Geometry: final body of the model. Coordinates: model frame, mm. Give positions to 0.01 mm unless a question says otherwise; leave off trailing zeros. Write each loop counter-clockwise with the first axis right and the second up, starting at its lowest first coordinate (ties: lowest second). Pieces come first, ordered by that corner, then holes. Notation, with made-up numbers: (23.25, 29) -> (47.25, 29) arc R21 cw to (47.25, 51) -> close; hole circle Ø6 at (85.25, 69). An arc over 180 degrees is marked (long way). Answer as a JSON object with one key per item and string values. Group by question number.
(1) Draft query along Z for faces 1 (the face through (3.13, -37.68, -101.61)), 2 (the face through (0, -166, -142)). Return one class per face: +Z half, -Z half, draft (parallel to the pull), parting line (faces both ways), or undercut.
(2) Material intervals for probe 1 along Y at (x, z) = (6, -158) (3 decimals); probe 2 along Z at (x, y) = (3.75, -44.5); probe 3 along Y at (x, z) = (6.25, -164.5) (3 decimals), sorted ascending.
(3) Contact query for flat-ended pins moving along their axis: pin 1 Ø1.9 at (x, z) = (2, 2) entering from -Y; pin 2 Ø1 at (x, z) = (3, -233) entering from +Y; pin 3 Ø3 at (x, y) = (4, -81) entering from -Z. Output: stop coordinate, or through.
(4) Section query C-C on y = -83. Output: boundary loops of the cut face in (x, z), plus the area to 3 significant figures.
(5) Section query B-B on z = -266. Output: boundary loops of the cut face in (x, y), plus the area to 3 significant figures.
(6) Section query A-A on x = 2.25. State how many separate pieces and enclosed holes the cut face has, plus the area to 3 significant figures.
from build123d import *

# Parameters (mm, degrees)
SKETCH1_R           = 9.525
SKETCH1_W           = 12.573
SKETCH1_H           = 6.35
BOSS_EXTRUDE1_DEPTH = 6.35


with BuildPart() as part:
    # Sketch1 → Boss-Extrude1 (new body)
    with BuildSketch(Plane(origin=(0, 0, 0), x_dir=(0, 0, -1), z_dir=(1, 0, 0))):
        Polygon((0, 0), (6.223, 0), (6.223, 6.35), (19.177, 6.35), (19.177, 0), (260.223, 0), (260.223, 6.35), (273.177, 6.35), (273.177, 0), (279.4, 0), (279.4, -12.573), (285.75, -12.573), (285.75, -25.527), (279.4, -25.527), (279.4, -37.973), (285.75, -37.973), (285.75, -50.927), (279.4, -50.927), (279.4, -63.373), (285.75, -63.373), (285.75, -76.327), (279.4, -76.327), (279.4, -88.773), (285.75, -88.773), (285.75, -101.727), (279.4, -101.727), (279.4, -114.173), (285.75, -114.173), (285.75, -127.127), (279.4, -127.127), (279.4, -139.573), (285.75, -139.573), (285.75, -152.527), (279.4, -152.527), (279.4, -164.973), (285.75, -164.973), (285.75, -177.927), (279.4, -177.927), (279.4, -190.373), (285.75, -190.373), (285.75, -203.327), (279.4, -203.327), (279.4, -215.773), (285.75, -215.773), (285.75, -228.727), (279.4, -228.727), (279.4, -241.173), (285.75, -241.173), (285.75, -254.127), (279.4, -254.127), (279.4, -266.573), (285.75, -266.573), (285.75, -279.527), (279.4, -279.527), (279.4, -291.973), (285.75, -291.973), (285.75, -304.927), (279.4, -304.927), (279.4, -317.373), (285.75, -317.373), (285.75, -330.327), (279.4, -330.327), (279.4, -342.9), (272.923, -342.9), (272.923, -336.55), (260.477, -336.55), (260.477, -342.9), (247.523, -342.9), (247.523, -336.55), (235.077, -336.55), (235.077, -342.9), (222.123, -342.9), (222.123, -336.55), (209.677, -336.55), (209.677, -342.9), (196.723, -342.9), (196.723, -336.55), (184.277, -336.55), (184.277, -342.9), (171.323, -342.9), (171.323, -336.55), (158.877, -336.55), (158.877, -342.9), (145.923, -342.9), (145.923, -336.55), (133.477, -336.55), (133.477, -342.9), (120.523, -342.9), (120.523, -336.55), (108.077, -336.55), (108.077, -342.9), (95.123, -342.9), (95.123, -336.55), (82.677, -336.55), (82.677, -342.9), (69.723, -342.9), (69.723, -336.55), (57.277, -336.55), (57.277, -342.9), (44.323, -342.9), (44.323, -336.55), (31.877, -336.55), (31.877, -342.9), (18.923, -342.9), (18.923, -336.55), (6.477, -336.55), (6.477, -342.9), (0, -342.9), (0, -330.327), (-6.35, -330.327), (-6.35, -317.373), (0, -317.373), (0, -304.927), (-6.35, -304.927), (-6.35, -291.973), (0, -291.973), (0, -279.527), (-6.35, -279.527), (-6.35, -266.573), (0, -266.573), (0, -254.127), (-6.35, -254.127), (-6.35, -241.173), (0, -241.173), (0, -228.727), (-6.35, -228.727), (-6.35, -215.773), (0, -215.773), (0, -203.327), (-6.35, -203.327), (-6.35, -190.373), (0, -190.373), (0, -177.927), (-6.35, -177.927), (-6.35, -164.973), (0, -164.973), (0, -152.527), (-6.35, -152.527), (-6.35, -139.573), (0, -139.573), (0, -127.127), (-6.35, -127.127), (-6.35, -114.173), (0, -114.173), (0, -101.727), (-6.35, -101.727), (-6.35, -88.773), (0, -88.773), (0, -76.327), (-6.35, -76.327), (-6.35, -63.373), (0, -63.373), (0, -50.927), (-6.35, -50.927), (-6.35, -37.973), (0, -37.973), (0, -25.527), (-6.35, -25.527), (-6.35, -12.573), (0, -12.573), align=None)
        with Locations((111.125, -38.1)):
            Circle(SKETCH1_R, mode=Mode.SUBTRACT)
        with Locations((168.275, -38.1)):
            Circle(SKETCH1_R, mode=Mode.SUBTRACT)
        with Locations((127, -137.16)):
            Rectangle(SKETCH1_W, SKETCH1_H, mode=Mode.SUBTRACT)
        with Locations((152.4, -137.16)):
            Rectangle(SKETCH1_W, SKETCH1_H, mode=Mode.SUBTRACT)
    extrude(amount=BOSS_EXTRUDE1_DEPTH)


solid = part.part
Answer list:
{
 "1": {"face 1": "undercut", "face 2": "draft"},
 "2": {"probe 1": "-342.9 to -140.335, -133.985 to 0", "probe 2": "-285.75 to -175.33, -161.22 to -118.18, -104.07 to 6.35", "probe 3": "-336.55 to -46.845, -29.355 to 0"},
 "3": {"pin 1": "y = -330.33", "pin 2": "y = 0", "pin 3": "z = -279.4"},
 "4": {"outline": "(0, -279.4) -> (6.35, -279.4) -> (6.35, 0) -> (0, 0) -> close", "area": "1,770 mm2"},
 "5": {"outline": "(0, -336.55) -> (6.35, -336.55) -> (6.35, 6.35) -> (0, 6.35) -> close", "area": "2,180 mm2"},
 "6": {"separate pieces": "1", "enclosed holes": "4", "area": "96,500 mm2"}
}
